```python
from build123d import *

# Parameters (mm, degrees)
F0_W     = 50.5277775228
F0_H     = 38.6841930449
F1_DEPTH = 74.168
F2_T     = -2.54
F3_R     = 9.0198311592
F4_DEPTH = 71.882


with BuildPart() as f1:
    # F0 (on Top) → F1 (new body)
    with BuildSketch(Plane.XY):
        with Locations((25.2638887614, -19.3420965225)):
            Rectangle(F0_W, F0_H)
    extrude(amount=F1_DEPTH)

    # F2
    f2_openings = [f1.faces().sort_by_distance(p)[0] for p in [
        (25.263889, -19.342097, 74.168),
    ]]
    offset(amount=F2_T, openings=f2_openings)

    # F3 (on face) → F4 (cut)
    with BuildSketch(Plane.XZ.offset(38.6841930449)):
        with Locations((24.6360246092, 41.1775447428)):
            Circle(F3_R)
    extrude(amount=-F4_DEPTH, mode=Mode.SUBTRACT)


solid = f1.part
```
Could you check a few things on this model? Use its own coordinates, in mm. A direction names the side the tool comes from. Coordinates: 2 decimals unless noted, no trailing zeros. Order: outer loops, then holes, each group sorted by start corner. A loop starts at its lowest first (then second) coordinate and runs counter-clockwise, first axis right, second up. Notation, with made-up numbers: M 31,27 L 46,27 A14 ccw 46,43 Z; hole C -19.75,81 d11. An arc over 180 degrees is marked long. Use one line per item in the form item = value. Start each with the question number.
1. For pin 1 (1.5 mm diameter, centred on x = 27.5, y = -11.5, fed in from +Z), with a flat end and sliding along its axis, tell me the tip position at first contact or that it passes through.
2. On a 3-axis mill with a long thin cutter (end or side, diameter ignored), from which of +Z, -Z, +X, -X, +Y, -Y can I reach the whole of each face in a straight line? I mean faces 1 (the flat face through (50.528, -20, 37)), 2 (the flat face through (25, -19, 2.54)). Say none if no direction works.
3. Suppose I cut it at D-D on z = 28. Write out the boundary of the cut face in (x, y).
4. We'd pull the mould along Z, two halves only. Please class faces 3 (the flat face through (23.3, -36.4, 74.168)), 4 (the cylindrical face through (22.681, -37.432, 32.372)), 5 (the flat face through (25, -38.684, 28)): +Z half, -Z half, draft (parallel to the pull), parting line (faces both ways), or undercut.
5. Suppose I cut it at B-B on x = 44.5. Write out the boundary of the cut face in (y, z).
6. Suppose I cut it at A-A on z = 48.5. Write out the boundary of the cut face in (x, y), then the cut area to 3 significant figures.
7. Please list where these lines run through material, in increasing order: line 1 (Y direction, x = 29.5, z = 61.5); line 2 (X direction, y = -9.5, z = 49); line 3 (Z direction, x = 18.5, y = -10).
8. Suppose I cut it at C-C on y = -33. Write out the boundary of the cut face in (x, z).
Geometry says:
q1.pin_1 = 2.54
q2.face_1 = +Z, -Z, +X, +Y, -Y
q2.face_2 = +Z
q3.outline = M 0,-38.68 L 50.53,-38.68 L 50.53,0 L 0,0 Z; hole M 2.54,-36.14 L 47.99,-36.14 L 47.99,-2.54 L 2.54,-2.54 Z
q4.face_3 = +Z half
q4.face_4 = undercut
q4.face_5 = draft
q5.outline = M -38.68,0 L 0,0 L 0,74.17 L -2.54,74.17 L -2.54,2.54 L -36.14,2.54 L -36.14,74.17 L -38.68,74.17 Z
q6.outline = M 0,-38.68 L 19.37,-38.68 L 19.37,-36.14 L 2.54,-36.14 L 2.54,-2.54 L 19.37,-2.54 L 19.37,0 L 0,0 Z; M 29.9,-38.68 L 50.53,-38.68 L 50.53,0 L 29.9,0 L 29.9,-2.54 L 47.99,-2.54 L 47.99,-36.14 L 29.9,-36.14 Z
q6.area = 374 mm^2
q7.line_1 = -38.68 to -36.14, -2.54 to 0
q7.line_2 = 0 to 2.54, 47.99 to 50.53
q7.line_3 = 0 to 2.54
q8.outline = M 0,0 L 50.53,0 L 50.53,74.17 L 47.99,74.17 L 47.99,2.54 L 2.54,2.54 L 2.54,74.17 L 0,74.17 Z
